Autodesk Inventor part; units mm, degrees
ref_plane "YZ Plane" through (0, 0, 0) normal (1, 0, 0) x (0, 1, 0)
ref_plane "XZ Plane" through (0, 0, 0) normal (0, 1, 0) x (-1, 0, 0)
ref_plane "XY Plane" through (0, 0, 0) normal (0, 0, 1) x (1, 0, 0)
sketch "Sketch2" plane through (0, 0, 0) normal (1, 0, 0) x (0, 1, 0)
  line L0 (0, 0) -> (0, -31.496)
  line L1 (0, -31.496) -> (41.275, -31.496)
  line L2 (41.275, -31.496) -> (41.275, 0)
  line L3 (41.275, 0) -> (0, 0)
  dimension "d0" = 41.275
  dimension "d2" = 31.496
revolve "Revolution1" add sketch "Sketch2" angle 360 about axis through (0, 41.275, 0) along (0, -1, 0)
chamfer "Chamfer1" distance 1.27 angle 45 2 edges at (0, 41.275, 31.496) (0, 0, 31.496)
sketch "Sketch4" plane through (0, 0, 0) normal (0, -1, 0) x (1, 0, 0)
  circle A0 centre (0, 0) radius 3.175
  point P0 (0, 0)
hole "Hole2" at (0, 0, 0) direction (0, 1, 0) diameter 3.302 depth 10.922 tip angle 118
sketch "Sketch5" plane through (0, 41.275, 0) normal (0, 1, 0) x (1, 0, 0)
  circle A0 centre (0, 0) radius 1.651
  point P0 (0, 0)
hole "Hole3" at (0, 41.275, 0) direction (0, -1, 0) diameter 3.9624 depth 10.922 tip angle 118
properties part number "Fixture_Weight"
For this review, take the finished solid that the model builds, in its own axes (mm). A direction names the side the tool comes from. Give positions to 0.01 mm unless a question says otherwise; leave off trailing zeros. Order: outer loops, then holes, each group sorted by start corner. A loop starts at its lowest first (then second) coordinate and runs counter-clockwise, first axis right, second up.
1) Wall thickness on line 1 (X direction, y = 37, z = 0); line 2 (X direction, y = 6, z = 0); line 3 (Z direction, x = -12, y = 27): over which ranges is each line inside the solid? List them lowest first.
2) Take a section at A-A (y = 15.5). Give the boundary of the cut face in (x, z), then the cut area to 3 significant figures.
3) For faces 1 (the face through (0.632, 5.537, -1.525)), 2 (the face through (-1.964, 35.738, -0.258)), 3 (the face through (0, 41.275, -6)), list the 3-axis set-ups (+Z, -Z, +X, -X, +Y, -Y) from which the entire face can be reached by the end or side of a thin tool; tool diameter is ignored.
4) Insertion check: pin 1 (8 mm diameter, centred on y = 8, z = -16.5, fed in from -X); pin 2 (3 mm diameter, centred on x = -12.5, y = 6, fed in from +Z); pin 3 (8 mm diameter, centred on x = -16, y = 5, fed in from -Z). Each pin has a flat end and moves straight along its axis. Give the tip position at first contact, or say it passes through.
5) The part is to be moulded in two halves that separate along X. For faces 4 (the face through (30.747, 20.909, 6.828)), 5 (the face through (0, 0, -6)), 6 (the face through (0.1, 29.37, 0.33)), say which applies: released by +X, released by -X, zero draft, split by the parting line, or undercut.
Derived:
1. line 1: x = -31.5 to -1.98, 1.98 to 31.5
1. line 2: x = -31.5 to -1.65, 1.65 to 31.5
1. line 3: z = -29.12 to 29.12
2. outline: circle Ø62.99 at (0, 0)
2. area: 3,120 mm2
3. face 1: -Y
3. face 2: +Y
3. face 3: +Z, -Z, +X, -X, +Y
4. pin 1: stops at x = -28.91
4. pin 2: stops at z = 29.51
4. pin 3: stops at z = -29.12
5. face 4: split by the parting line
5. face 5: zero draft
5. face 6: undercut
